For this review, take the finished solid that the model builds, in its own axes (mm). Give positions to 0.01 mm unless a question says otherwise; leave off trailing zeros. Write each loop counter-clockwise with the first axis right and the second up, starting at its lowest first coordinate (ties: lowest second). Pieces come first, ordered by that corner, then holes. Notation, with made-up numbers: (67.5, 31) -> (114.5, 31) arc R19 ccw to (114.5, 64) -> close; hole circle Ø6 at (63, -19). An arc over 180 degrees is marked (long way). Answer as CSV lines item,"result".
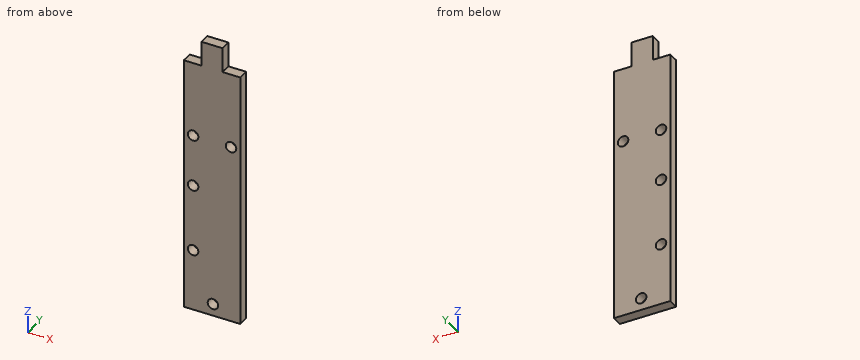
Autodesk Inventor part; units mm, degrees
ref_plane "YZ Plane" through (0, 0, 0) normal (1, 0, 0) x (0, 1, 0)
ref_plane "XZ Plane" through (0, 0, 0) normal (0, 1, 0) x (-1, 0, 0)
ref_plane "XY Plane" through (0, 0, 0) normal (0, 0, 1) x (1, 0, 0)
ref_plane "Work Plane1" through (0, 0, 0) normal (0, 0, 1) x (1, 0, 0)
sketch "Sketch1" plane through (0, 0, 0) normal (0, 0, 1) x (1, 0, 0)
  line L0 (88.5744, 66.01) -> (72.4744, 66.01)
  line L1 (72.4744, 66.01) -> (88.5744, 66.01)
  line L2 (88.5744, 66.01) -> (88.5744, 63.01)
  line L3 (88.5744, 63.01) -> (72.4744, 63.01)
  line L4 (72.4744, 63.01) -> (72.4744, 66.01)
  point P0 (0, 0)
  dimension "d0" = 3
extrude "Extrusion1" add sketch "Sketch1" against normal blind 80
sketch "Sketch2" plane through (72.4744, 66.01, 0) normal (0, 1, 0) x (1, 0, 0)
  circle A0 centre (2.65, 28.5) radius 1.5
  circle A1 centre (13.45, 28.5) radius 1.5
  circle A2 centre (2.65, 43.3) radius 1.5
  circle A3 centre (2.65, 62.4) radius 1.5
  point P0 (-72.4744, 0)
extrude "Extrusion2" cut sketch "Sketch2" against normal blind 80
ref_plane "Work Plane2" through (0, 0, 0) normal (0, 0, 1) x (1, 0, 0)
sketch "Sketch3" plane through (0, 0, 0) normal (0, 0, 1) x (1, 0, 0)
  point P0 (0, 0)
sketch "Sketch4" plane through (72.4744, 66.01, 0) normal (0, 1, 0) x (1, 0, 0)
  line L0 (0, 0) -> (16.1, 0)
  line L1 (5, 0) -> (11, 0)
  line L2 (11, 0) -> (11, 7.0573)
  line L3 (11, 7.0573) -> (5, 7.0573)
  line L4 (5, 7.0573) -> (5, 0)
  line L5 (0, 0) -> (0, 80)
  line L6 (0, 0) -> (0, 80)
  line L7 (0, 0) -> (16.1, 0)
  line L8 (16.1, 0) -> (16.1, 7.0573)
  line L9 (16.1, 7.0573) -> (0, 7.0573)
  line L10 (0, 7.0573) -> (0, 0)
  point P0 (-72.4744, 0)
  point P1 (11, 7.0573)
  point P2 (11, 0)
  point P3 (5, 7.0573)
  dimension "d5" = 6
  dimension "d6" = 5
extrude "Extrusion3" cut sketch "Sketch4" against normal blind 80 contours L5 L9 L4 L0 | L2 L9 L8 L0
sketch "Sketch5" plane through (72.4744, 66.01, -80) normal (0, 1, 0) x (1, 0, 0)
  circle A0 centre (8.3144, -3.4296) radius 1.5
  point P0 (-72.4744, -80)
  dimension "d9" = 3
extrude "Extrusion4" cut sketch "Sketch5" against normal blind 80
properties part number "thanhdolimit"
Q1. Add section A-A (z = -62.4). Write out the cut boundary in (x, y).
Answer block:
outline,"(72.47, 63.01) -> (73.62, 63.01) -> (73.62, 66.01) -> (72.47, 66.01) -> close; (76.62, 63.01) -> (88.57, 63.01) -> (88.57, 66.01) -> (76.62, 66.01) -> close"
Q2. Clearance check with flat-ended pins moving along their axes: pin 1 (0.9 mm diameter, centred on y = 64.5, z = -4, fed in from -X); pin 2 (2.5 mm diameter, centred on x = 75.12, z = -43.3, fed in from -Y) (3 decimals); pin 3 (1.5 mm diameter, centred on x = 74, y = 64, fed in from +Z). State where each tip first meets the part, or that it passes through.
Answer block:
pin 1,"stops at x = 77.47"
pin 2,"passes through"
pin 3,"stops at z = -7.06"
Q3. Add section B-B (z = -28.5). Write out the cut boundary in (x, y).
Answer block:
outline,"(72.47, 63.01) -> (73.62, 63.01) -> (73.62, 66.01) -> (72.47, 66.01) -> close; (76.62, 63.01) -> (84.42, 63.01) -> (84.42, 66.01) -> (76.62, 66.01) -> close; (87.42, 63.01) -> (88.57, 63.01) -> (88.57, 66.01) -> (87.42, 66.01) -> close"
Q4. Add section C-C (y = 64.7). Write out the cut boundary in (x, z), plus the area to 3 significant figures.
Answer block:
outline,"(72.47, -80) -> (88.57, -80) -> (88.57, -7.06) -> (83.47, -7.06) -> (83.47, 0) -> (77.47, 0) -> (77.47, -7.06) -> (72.47, -7.06) -> close; hole circle Ø3 at (75.12, -62.4); hole circle Ø3 at (75.12, -43.3); hole circle Ø3 at (75.12, -28.5); hole circle Ø3 at (80.79, -76.57); hole circle Ø3 at (85.92, -28.5)"
area,"1,180 mm2"
Q5. To check wall thickness, follow probe 1 along X at (y, z) = (65.25, -28.5); probe 2 along Z at (x, y) = (76.5, 63.75); probe 3 along Z at (x, y) = (85.75, 65.55). State the ranges of each line that lie inside material, in increasing order. Write a range as [from, to].
Answer block:
probe 1,"x = [72.47, 73.62], [76.62, 84.42], [87.42, 88.57]"
probe 2,"z = [-80, -63], [-61.8, -43.9], [-42.7, -29.1], [-27.9, -7.06]"
probe 3,"z = [-80, -29.99], [-27.01, -7.06]"
